Design review of the part built by this model. Coordinates are the model's own, in mm. Face numbers are marked on the shaded views. A direction names the side the tool comes from. Round coordinates to 2 decimals unless told otherwise and drop trailing zeros. Write each loop counter-clockwise with the first axis right and the second up, starting at its lowest first coordinate (ties: lowest second). Pieces come first, ordered by that corner, then holes. Notation, with made-up numbers: (52, -33) -> (79, -33) arc R30 ccw to (79, 2) -> close; hole circle Ø6 at (42.25, -20). An arc over 180 degrees is marked (long way). One line per question, with ' | ' between items. Start each with the question number.
1) For the marked faces 1, 2 and 3, list the 3-axis set-ups (+Z, -Z, +X, -X, +Y, -Y) from which the entire face can be reached by the end or side of a thin tool; tool diameter is ignored.
2) Mouldability with a two-part tool opening along Y and no side actions: class the marked faces 4, 5 and 6 as +Y half, -Y half, draft (parallel to the pull), parting line (faces both ways), or undercut.
3) Insertion check: pin 1 Ø4 at (x, z) = (32.5, 92.5) entering from -Y; pin 2 Ø6 at (x, z) = (-27.5, 24) entering from -Y; pin 3 Ø2 at (x, z) = (36.5, 174.5) entering from +Y. Each pin has a flat end and moves straight along its axis. Give the tip position at first contact, or say it passes through.
4) Consider section A-A (z = 25.4). Give the boundary of the cut face in (x, y).
5) For probe 1 along Z at (x, y) = (0, -17.5); probe 2 along Z at (x, y) = (0, -30); probe 3 along Z at (x, y) = (34, -2.5), list the stretches that pass through material, from the lowest coordinate up.
6) Consider section C-C (x = -17). Count the separate pieces of the cut face and the enclosed holes in it, then the cut area to 3 significant figures.
7) Consider section B-B (z = 158). Give the boundary of the cut face in (x, y).
```python
from build123d import *

# Parameters (mm, degrees)
F1_DEPTH  = 203.2
F2_R      = 13.97
F3_DEPTH  = 101.601
F4_R      = 13.97
F5_DEPTH  = 101.6
F6_R      = 13.97
F7_DEPTH  = 101.601
F8_R      = 13.97
F9_DEPTH  = 122.64304911
F11_DEPTH = 101.6010001
F12_R     = 12.7
F13_DEPTH = 25.4
F15_DEPTH = 122.64304911
F16_R     = 12.7
F17_DEPTH = 25.4


with BuildPart() as f1:
    # F0 (on Top) → F1 (new body)
    with BuildSketch(Plane.XY):
        Polygon((-21.0420489686, -50.8), (21.0420489686, -50.8), (50.8, -21.0420489686), (50.8, 21.0420489686), (21.0420489686, 50.8), (-21.0420489686, 50.8), (-50.8, 21.0420489686), (-50.8, -21.0420489686), align=None)
    extrude(amount=F1_DEPTH)

    # F2 (on face) → F3 (cut, through all)
    with BuildSketch(Plane.XZ.offset(50.8)):
        with Locations((0, 25.4)):
            Circle(F2_R)
    extrude(amount=-F3_DEPTH, mode=Mode.SUBTRACT)

    # F4 (on face) → F5 (cut)
    with BuildSketch(Plane(origin=(35.9210244843, -35.9210244843, 0), x_dir=(0.7071067812, 0.7071067812, 0), z_dir=(0.7071067812, -0.7071067812, 0))):
        with Locations((0, 50.8)):
            Circle(F4_R)
    extrude(amount=-F5_DEPTH, mode=Mode.SUBTRACT)

    # F6 (on face) → F7 (cut, through all)
    with BuildSketch(Plane.YZ.offset(50.8)):
        with Locations((0, 76.2)):
            Circle(F6_R)
    extrude(amount=-F7_DEPTH, mode=Mode.SUBTRACT)

    # F8 (on face) → F9 (cut, through all)
    with BuildSketch(Plane(origin=(35.9210244843, 35.9210244843, 0), x_dir=(-0.7071067812, 0.7071067812, 0), z_dir=(0.7071067812, 0.7071067812, 0))):
        with Locations((0, 101.6)):
            Circle(F8_R)
    extrude(amount=-F9_DEPTH, mode=Mode.SUBTRACT)

    # F10 (on face) → F11 (cut, through all)
    with BuildSketch(Plane.XZ.offset(50.8)):
        Polygon((50.8, 152.4), (50.8, 203.2), (40.0646968374, 163.1353031626), align=None)
    extrude(amount=-F11_DEPTH, mode=Mode.SUBTRACT)

    # F12 (on face) → F13 (cut)
    with BuildSketch(Plane(origin=(-3.4029547439, 0, 0.9118189755), x_dir=(0, 1, 0), z_dir=(0.9659258263, 0, -0.2588190451))):
        with Locations((0, 184.0241353931)):
            Circle(F12_R)
    extrude(amount=-F13_DEPTH, mode=Mode.SUBTRACT)

    # F14 (on face) → F15 (cut, through all)
    with BuildSketch(Plane(origin=(35.9210244843, 35.9210244843, 0), x_dir=(-0.7071067812, 0.7071067812, 0), z_dir=(0.7071067812, 0.7071067812, 0))):
        Polygon((50.8, 152.4), (50.8, 203.2), (42.1126883595, 153.931807432), align=None)
    extrude(amount=-F15_DEPTH, mode=Mode.SUBTRACT)

    # F16 (on face) → F17 (cut)
    with BuildSketch(Plane(origin=(-10.2664451766, 10.2664451766, -2.5600819123), x_dir=(-0.6756735354, -0.717688543, -0.1684886606), z_dir=(-0.6963642403, 0.6963642403, -0.1736481777))):
        with Locations((-31.4004860543, 180.8281922458)):
            Circle(F16_R)
    extrude(amount=-F17_DEPTH, mode=Mode.SUBTRACT)


solid = f1.part
```
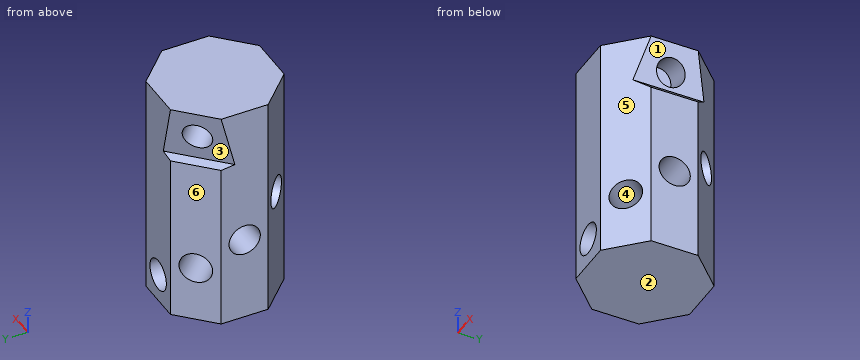
From the geometry:
1) face 1: +X, +Y, -Y | face 2: -Z, +X, -X, +Y, -Y | face 3: -X, +Y
2) face 4: undercut | face 5: -Y half | face 6: +Y half
3) pin 1: stops at y = -41.34 | pin 2: stops at y = -47.34 | pin 3: stops at y = 36.34
4) outline: (-50.8, -21.04) -> (-21.04, -50.8) -> (-13.97, -50.8) -> (-13.97, 50.8) -> (-21.04, 50.8) -> (-50.8, 21.04) -> close; (13.97, -50.8) -> (21.04, -50.8) -> (50.8, -21.04) -> (50.8, 21.04) -> (21.04, 50.8) -> (13.97, 50.8) -> close
5) probe 1: z = 0 to 11.43, 39.37 to 44.32, 57.28 to 95.12, 108.08 to 203.2 | probe 2: z = 0 to 11.43, 39.37 to 203.2 | probe 3: z = 0 to 62.46, 89.94 to 168.51, 194.3 to 203.2
6) separate pieces: 1 | enclosed holes: 4 | area: 17,700 mm2
7) outline: (-50.8, -21.04) -> (-21.04, -50.8) -> (21.04, -50.8) -> (45.2, -26.64) -> (45.2, 26.64) -> (21.04, 50.8) -> (-9.77, 50.8) -> (-50.8, 9.77) -> close
